```python
from build123d import *

# Parameters (mm, degrees)
HOLE_WIZARD_M5_2_D               = 4.2
HOLE_WIZARD_M5_2_DEPTH           = 15
HOLE_WIZARD_M5_2_ON_FACE_2_D     = 4.2
HOLE_WIZARD_M5_2_ON_FACE_2_DEPTH = 15


with BuildPart() as part:
    # 草图1 → 旋转1 (revolve)
    with BuildSketch(Plane.XY, mode=Mode.PRIVATE) as revolve_1_sk:
        Polygon((4, 30.2), (15, 30.2), (15, 18.7), (10.25, 16.525), (10.25, 13.525), (15, 11.35), (15, 9.35), (10.25, 7.175), (10.25, 4.175), (15, 2), (15, 0), (4, 0), align=None)
    revolve(revolve_1_sk.sketch.rotate(Axis((0, 48.963970588, 0), (0, -1, 0)), 90), axis=Axis((0, 48.963970588, 0), (0, -1, 0)))

    # M5 螺纹孔2
    with Locations(Plane(origin=(15, 24.45, 0), x_dir=(0, 0, 1), z_dir=(1, 0, 0))):
        with Locations((0, 0)):
            Hole(HOLE_WIZARD_M5_2_D / 2, depth=HOLE_WIZARD_M5_2_DEPTH)

    # M5 螺纹孔2 on face 2
    with Locations(Plane(origin=(0, 24.45, 15), x_dir=(1, 0, 0), z_dir=(0, 0, 1))):
        with Locations((0, 0)):
            Hole(HOLE_WIZARD_M5_2_ON_FACE_2_D / 2, depth=HOLE_WIZARD_M5_2_ON_FACE_2_DEPTH)


solid = part.part
```
Build history of the part. All positions in model axes, mm. A direction names the side the tool comes from. Give positions to 0.01 mm unless a question says otherwise; leave off trailing zeros. Loops run counter-clockwise (first coordinate to the right, second up) from the corner with the lowest first, then second, coordinate; pieces in that order, holes last.
Item 1: Drill centre lines: line 1 (Y direction, x = -10, z = -8); line 2 (Y direction, x = 5, z = 13.5); line 3 (Z direction, x = 11, y = 24). Where is each one in solid material? Low to high.
Answers follow:
line 1: y = 0 to 3, 8.35 to 12.35, 17.7 to 30.2
line 2: y = 0 to 2.28, 9.07 to 11.63, 18.42 to 30.2
line 3: z = -10.2 to -2.05, 2.05 to 10.2
Item 2: Slice it at B-B, the plane x = 0. List the corners of the cut face in (y, z) (3 decimals).
Answers follow:
outline: (0, -15) - (2, -15) - (4.175, -10.25) - (7.175, -10.25) - (9.35, -15) - (11.35, -15) - (13.525, -10.25) - (16.525, -10.25) - (18.7, -15) - (30.2, -15) - (30.2, -4) - (0, -4) - close; (0, 4) - (22.35, 4) - (22.35, 15) - (18.7, 15) - (16.525, 10.25) - (13.525, 10.25) - (11.35, 15) - (9.35, 15) - (7.175, 10.25) - (4.175, 10.25) - (2, 15) - (0, 15) - close; (26.55, 4) - (30.2, 4) - (30.2, 15) - (26.55, 15) - close
Item 3: Slice it at A-A, the plane z = 0. List the corners of the cut face in (x, y) (3 decimals), and give its area (3 significant figures).
Answers follow:
outline: (-15, 0) - (-4, 0) - (-4, 30.2) - (-15, 30.2) - (-15, 18.7) - (-10.25, 16.525) - (-10.25, 13.525) - (-15, 11.35) - (-15, 9.35) - (-10.25, 7.175) - (-10.25, 4.175) - (-15, 2) - close; (4, 0) - (15, 0) - (15, 2) - (10.25, 4.175) - (10.25, 7.175) - (15, 9.35) - (15, 11.35) - (10.25, 13.525) - (10.25, 16.525) - (15, 18.7) - (15, 22.35) - (4, 22.35) - close; (4, 26.55) - (15, 26.55) - (15, 30.2) - (4, 30.2) - close
area: 520 mm2
Item 4: Which spindle directions (+Z, -Z, +X, -X, +Y, -Y) get a long thin tool onto all of the face, cutting with end or side? Do faces 4 (the face through (3, 30.2, -3)), 5 (the face through (3.926, 5.654, 9.468)). Say none if no direction does.
Answers follow:
face 4: +Z, -Z, +X, -X, +Y
face 5: none
Item 5: Slice it at C-C, the plane y = 26. List the corners of the cut face in (x, z), and give its area (3 significant figures).
Answers follow:
outline: (-1.42, 3.74) - (-1.42, 14.93) arc R15 ccw (long way) to (14.93, -1.42) - (3.74, -1.42) arc R4 cw (long way) to start; (1.42, 3.74) arc R4 cw to (3.74, 1.42) - (14.93, 1.42) arc R15 ccw to (1.42, 14.93) - close
area: 594 mm2
Item 6: Flat gauge pins, fed straight in: pin 1 (1 mm diameter, centred on x = 10.5, z = 11, fed in from -Y); pin 2 (2 mm diameter, centred on y = 23.5, z = 1.5, fed in from -X); pin 3 (1 mm diameter, centred on x = 6.5, y = 27, fed in from -Z); pin 4 (2 mm diameter, centred on y = 26, z = 7.5, fed in from -X). Where does each tip first touch, or does it go through?
Answers follow:
pin 1: stops at y = 0
pin 2: stops at x = -14.99
pin 3: stops at z = -13.75
pin 4: stops at x = -13.52
Item 7: Pull direction Z, two halves, no side cores. Call faces 1 (the face through (-2.003, 25.081, 9.121)), 2 (the face through (-12.65, 24.37, 8.06)), 3 (the face through (9.12, 25.25, -1.94)): released by +Z, released by -Z, zero draft, split by the parting line, or undercut.
Answers follow:
face 1: zero draft
face 2: split by the parting line
face 3: undercut
Item 8: Slice it at D-D, the plane x = 11.5. Give the number of separate pieces and of enclosed holes in the cut face, and give its area (3 significant figures).
Answers follow:
separate pieces: 3
enclosed holes: 1
area: 365 mm2
